Source: CAD feature listing. Evaluate the final solid. Frame: model axes, mm. Give positions to 0.01 mm unless a question says otherwise; leave off trailing zeros. Order: outer loops, then holes, each group sorted by start corner. A loop starts at its lowest first (then second) coordinate and runs counter-clockwise, first axis right, second up.
1) Material intervals for line 1 (Y direction, x = 123, z = 2.5); line 2 (Y direction, x = 50.5, z = 0.9); line 3 (X direction, y = 42.5, z = 2.1), sorted ascending.
2) Section D-D, the plane y = 32. Return loops of the section in (x, z), plus the area to 3 significant figures.
3) Section B-B, the plane z = 0.8. Return loops of the section in (x, y) (3 decimals).
4) Section A-A, the plane x = 110. Return loops of the section in (y, z), plus the area to 3 significant figures.
5) First-contact query: P1, Ø1.5, axis at x = 88.5, z = 4, coming from the -Y side. Flat tip, straight axial feed; report the tip coordinate or a pass-through.
6) Section C-C, the plane y = 47.5. Return loops of the section in (x, z).
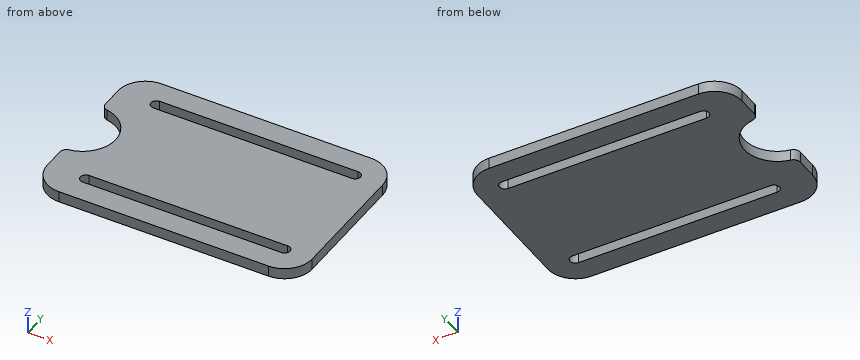
Autodesk Inventor part; units mm, degrees
ref_plane "YZ Plane" through (0, 0, 0) normal (1, 0, 0) x (0, 1, 0)
ref_plane "XZ Plane" through (0, 0, 0) normal (0, 1, 0) x (-1, 0, 0)
ref_plane "XY Plane" through (0, 0, 0) normal (0, 0, 1) x (1, 0, 0)
sketch "Sketch1" plane through (0, 0, 0) normal (0, 0, 1) x (1, 0, 0)
  line L0 (0, 0) -> (162.56, 0)
  line L1 (162.56, 0) -> (162.56, 81.28)
  line L2 (162.56, 81.28) -> (0, 81.28)
  line L3 (0, 81.28) -> (0, 0)
  dimension "d0" = 162.56
  dimension "d1" = 81.28
extrude "Extrusion1" add sketch "Sketch1" along normal blind 5.08
sketch "Sketch2" plane through (0, 0, 5.08) normal (0, 0, 1) x (1, 0, 0)
  line L0 (0, 0) -> (162.56, 0)
  line L1 (162.56, 0) -> (162.56, 81.28)
  line L2 (162.56, 81.28) -> (0, 81.28)
  line L3 (0, 81.28) -> (0, 0) construction
  line L4 (0, 40.64) -> (162.56, 40.64) construction
  arc A0 (40.64, 55.88) -> (40.64, 25.4) centre (40.64, 40.64) ccw construction
  arc A1 (78.3143, 55.88) -> (40.64, 81.28) centre (40.64, 40.64) ccw construction
  line L5 (0, 81.28) -> (0, 0)
  line L6 (0, 0) -> (162.56, 0)
  line L7 (0, 81.28) -> (40.64, 81.28) construction
  line L8 (162.56, 81.28) -> (162.56, 0)
  line L9 (162.56, 0) -> (40.64, 0)
  line L10 (0, 0) -> (0, 40.64)
  line L11 (0, 40.64) -> (0, 81.28)
  line L12 (40.64, 0) -> (0, 0) construction
  line L13 (40.64, 81.28) -> (162.56, 81.28)
  line L14 (40.64, 25.4) -> (78.3143, 25.4)
  line L15 (40.64, 55.88) -> (78.3143, 55.88)
  line L16 (162.56, 0) -> (162.56, 81.28)
  line L17 (162.56, 23.2866) -> (162.56, 55.88)
  line L18 (40.64, 25.4) -> (78.3143, 25.4)
  line L19 (162.56, 25.4) -> (162.56, 55.88) construction
  line L20 (162.56, 55.88) -> (40.64, 55.88)
  line L21 (40.64, 55.88) -> (40.64, 40.64) construction
  arc A2 (55.88, 40.64) -> (40.64, 55.88) centre (40.64, 40.64) ccw
  arc A3 (40.64, 25.4) -> (55.88, 40.64) centre (40.64, 40.64) ccw
  arc A4 (81.28, 40.64) -> (78.3143, 55.88) centre (40.64, 40.64) ccw construction
  arc A5 (78.3143, 25.4) -> (81.28, 40.64) centre (40.64, 40.64) ccw construction
  arc A6 (40.64, 81.28) -> (2.9657, 55.88) centre (40.64, 40.64) ccw construction
  arc A7 (40.64, 0) -> (78.3143, 25.4) centre (40.64, 40.64) ccw construction
  arc A8 (0, 40.64) -> (2.9657, 25.4) centre (40.64, 40.64) ccw
  arc A9 (2.9657, 25.4) -> (40.64, 0) centre (40.64, 40.64) ccw
  arc A10 (2.9657, 55.88) -> (0, 40.64) centre (40.64, 40.64) ccw
  line L22 (78.3143, 55.88) -> (162.56, 55.88)
  line L23 (78.3143, 25.4) -> (162.56, 25.4)
  line L24 (78.3143, 25.4) -> (162.56, 25.4)
  line L25 (40.64, 81.28) -> (40.64, 55.88)
  line L26 (40.64, 40.64) -> (40.64, 25.4) construction
  line L27 (40.64, 55.88) -> (40.64, 40.64) construction
  line L28 (40.64, 25.4) -> (40.64, 0)
  line L29 (40.64, 40.64) -> (40.64, 25.4)
  dimension "d4" = 30.48
extrude "Extrusion2" cut sketch "Sketch2" against normal blind 5.08 contours L28 L14 L23 L1 L0 | A3 A2 L15 L20 L1 L23 L14 | L2 L1 L20 L15 L25 keep common part
sketch "Sketch3" plane through (0, 0, 5.08) normal (0, 0, 1) x (1, 0, 0)
  line L0 (162.56, 0) -> (162.56, 81.28)
  line L1 (40.64, 0) -> (162.56, 0)
  line L2 (40.64, 40.64) -> (162.56, 40.64) construction
  line L3 (162.56, 40.64) -> (162.56, 25.4) construction
  line L4 (58.42, 68.58) -> (149.86, 68.58) construction
  line L5 (58.42, 66.08) -> (149.86, 66.08)
  line L6 (149.86, 71.08) -> (58.42, 71.08)
  arc A0 (58.42, 71.08) -> (58.42, 66.08) centre (58.42, 68.58) ccw
  arc A1 (149.86, 66.08) -> (149.86, 71.08) centre (149.86, 68.58) ccw
  line L7 (40.64, 55.88) -> (40.64, 81.28) construction
  line L8 (58.42, 12.7) -> (149.86, 12.7) construction
  line L9 (58.42, 15.2) -> (149.86, 15.2)
  line L10 (149.86, 10.2) -> (58.42, 10.2)
  arc A2 (58.42, 15.2) -> (58.42, 10.2) centre (58.42, 12.7) ccw
  arc A3 (149.86, 10.2) -> (149.86, 15.2) centre (149.86, 12.7) ccw
  line L11 (40.64, 0) -> (40.64, 25.4)
  line L12 (40.64, 55.88) -> (40.64, 81.28)
  arc A4 (40.64, 25.4) -> (40.64, 55.88) centre (40.64, 40.64) ccw
  line L13 (162.56, 81.28) -> (40.64, 81.28)
  point P0 (0, 0)
  point P1 (104.14, 68.58)
  point P2 (104.14, 12.7)
  dimension "d7" = 2.5
  dimension "d8" = 121.92
  dimension "d12" = 91.44
  dimension "d13" = 12.7
extrude "Extrusion3" cut sketch "Sketch3" against normal blind 5.08 contours A0 L6 A1 L5 | L9 A3 L10 A2
fillet "Fillet1" radius 12.7 2 edges at (162.56, 0, 2.54) (162.56, 81.28, 2.54)
fillet "Fillet2" radius 12.7 2 edges at (40.64, 81.28, 2.54) (40.64, 0, 2.54)
fillet "Fillet3" radius 3.175 2 edges at (40.64, 55.88, 2.54) (40.64, 25.4, 2.54)
equation "\"d0\" = 2 * d1"
equation "\"d13\" = d11"
equation "\"d11\" = 0.5 * d10"
properties part number "SuctionGrabberB" material "Wood (Birch)"
From the geometry:
1. line 1: y = 0 to 10.2, 15.2 to 66.08, 71.08 to 81.28
1. line 2: y = 0.32 to 29.02, 52.26 to 80.96
1. line 3: x = 55.77 to 162.56
2. outline: (53.19, 0) - (162.56, 0) - (162.56, 5.08) - (53.19, 5.08) - close
2. area: 556 mm2
3. outline: (40.64, 12.7) arc R12.7 ccw to (53.34, 0) - (149.86, 0) arc R12.7 ccw to (162.56, 12.7) - (162.56, 68.58) arc R12.7 ccw to (149.86, 81.28) - (53.34, 81.28) arc R12.7 ccw to (40.64, 68.58) - (40.64, 58.779) arc R3.175 ccw to (43.268, 55.652) arc R15.24 cw to (43.268, 25.628) arc R3.175 ccw to (40.64, 22.501) - close; hole (58.42, 10.2) - (149.86, 10.2) arc R2.5 ccw to (149.86, 15.2) - (58.42, 15.2) arc R2.5 ccw to start; hole (58.42, 66.08) - (149.86, 66.08) arc R2.5 ccw to (149.86, 71.08) - (58.42, 71.08) arc R2.5 ccw to start
4. outline: (0, 0) - (10.2, 0) - (10.2, 5.08) - (0, 5.08) - close; (15.2, 0) - (66.08, 0) - (66.08, 5.08) - (15.2, 5.08) - close; (71.08, 0) - (81.28, 0) - (81.28, 5.08) - (71.08, 5.08) - close
4. area: 362 mm2
5. P1: stops at y = 0
6. outline: (54.25, 0) - (162.56, 0) - (162.56, 5.08) - (54.25, 5.08) - close
